from build123d import *

# Parameters (mm, degrees)
SKETCH2_R = 0.75


with BuildPart() as part:
    # Sweep1: sweep along a path in Sketch1
    with BuildLine(Plane(origin=(0, 0, 0), x_dir=(0, 0, -1), z_dir=(1, 0, 0))) as sweep1_path:
        Line((41, 0), (33.5, 0))
        Line((33.5, 0), (33.5, -55))
        Line((33.5, -55), (0, -55))
        Line((0, -55), (0, 0))
        Line((0, 0), (-7.5, 0))
    # Sketch2 → Sweep1 (sweep)
    with BuildSketch(Plane.XY.offset(7.5)):
        Circle(SKETCH2_R)
    sweep(path=sweep1_path.line, transition=Transition.RIGHT)


solid = part.part
Design review of the part built by this model. Coordinates are the model's own, in mm. A direction names the side the tool comes from. Give positions to 0.01 mm unless a question says otherwise; leave off trailing zeros. Order: outer loops, then holes, each group sorted by start corner. A loop starts at its lowest first (then second) coordinate and runs counter-clockwise, first axis right, second up. Notation, with made-up numbers: (47.25, -35.5) - (52.25, -35.5) arc R29 cw to (52.25, -10.5) - close; hole circle Ø3 at (45.25, -33). An arc over 180 degrees is marked (long way). Write item = value, one per line. Start each with the question number.
Q1. Clearance check with flat-ended pins moving along their axes: pin 1 Ø5 at (y, z) = (-26, -35) entering from -X; pin 2 Ø10 at (y, z) = (-29.5, -23.5) entering from +X. State where each tip first meets the part, or that it passes through.
Q2. We need section A-A on y = 0. State the section outline as (x, z) points, plus the area to 3 significant figures.
Q3. Tool access review of faces 1 (the face through (0.403, -27.896, -32.868)), 2 (the face through (0, 0, 7.5)), 3 (the face through (-0.098, 0.744, 3.433)): name each direction out of +Z, -Z, +X, -X, +Y, -Y from which nothing blocks a thin tool from reaching the whole face with its end or side.
Q4. To check wall thickness, follow L1, parallel to Z at x = 0.1, y = -19.5; L2, parallel to Z at x = 0.5, y = -38; L3, parallel to Y at x = 0, z = -15. State the ranges of each line that lie inside material, in increasing order. Write a range as from..to.
Q5. We need section D-D on y = -31.5. State the section outline as (x, z) points.
Q6. Mouldability with a two-part tool opening along Z and no side actions: class faces 4 (the face through (0, 0, -41)), 5 (the face through (0.715, -27.104, -0.225)), 6 (the face through (-0.098, 0.744, -36.817)) as released by +Z, released by -Z, zero draft, split by the parting line, or undercut.
Q7. We need section B-B on x = 0. State the section outline as (y, z) points.
Q8. We need section C-C on z = -27.5. State the section outline as (x, y) points.
Working result:
q1.pin_1 = -0.75
q1.pin_2 = through
q2.outline = (-0.75, -41) - (0.75, -41) - (0.75, -33.5) arc R0.75 ccw to (-0.75, -33.5) - close; (-0.75, 0) arc R0.75 ccw to (0.75, 0) - (0.75, 7.5) - (-0.75, 7.5) - close
q2.area = 24.3 mm²
q3.face_1 = none
q3.face_2 = +Z, +X, -X, +Y, -Y
q3.face_3 = +Z
q4.L1 = -34.24..-32.76, -0.74..0.74
q4.L2 = -34.06..-32.94, -0.56..0.56
q4.L3 = -55.75..-54.25
q5.outline = circle Ø1.5 at (0, -33.5); circle Ø1.5 at (0, 0)
q6.face_4 = released by -Z
q6.face_5 = undercut
q6.face_6 = zero draft
q7.outline = (-55.75, -34.25) - (-0.75, -34.25) - (-0.75, -41) - (0.75, -41) - (0.75, -32.75) - (-54.25, -32.75) - (-54.25, -0.75) - (0.75, -0.75) - (0.75, 7.5) - (-0.75, 7.5) - (-0.75, 0.75) - (-55.75, 0.75) - close
q8.outline = circle Ø1.5 at (0, -55)
